```python
from build123d import *

# Parameters (mm, degrees)
SKETCH1_W                    = 200
SKETCH1_H                    = 70
BOSS_EXTRUDE1_DEPTH          = 150
CONVERT_SOLID1_START         = 1.36
CONVERT_SOLID1_DEPTH         = 197.28
CONVERT_SOLID1_START_2       = -1
CONVERT_SOLID1_2_DEPTH       = 202
CONVERT_SOLID1_3_DEPTH       = 2.184264069
CONVERT_SOLID1_START_3       = 198.815735931
CONVERT_SOLID1_4_DEPTH       = 2.184264069
CONVERT_SOLID1_START_4       = 1.184264069
CONVERT_SOLID1_5_DEPTH       = 197.631471862
CONVERT_SOLID1_6_DEPTH       = 0.175735931
CONVERT_SOLID1_START_5       = 198.64
CONVERT_SOLID1_7_DEPTH       = 0.175735931
CONVERT_SOLID1_START_6       = -68.815735931
CONVERT_SOLID1_8_DEPTH       = 67.631471862
CONVERT_SOLID1_9_DEPTH       = 0.175735931
CONVERT_SOLID1_START_7       = -1.36
CONVERT_SOLID1_10_DEPTH      = 0.175735931
EDGE_FLANGE1_STRIP_W         = 4.24
EDGE_FLANGE1_STRIP_H         = 0.76
EDGE_FLANGE1_STRIP_CUT_DEPTH = 148.269865
EDGE_FLANGE1_DEPTH           = 148.269865
MIRROR2_COPY_1_SKETCH_W      = 4.24
MIRROR2_COPY_1_SKETCH_H      = 0.76
MIRROR2_COPY_1_DEPTH         = 148.269865
MIRROR2_COPY_2_DEPTH         = 148.269865


with BuildPart() as part:
    # Sketch1 → Boss-Extrude1 (new body)
    with BuildSketch(Plane(origin=(0, 0, 0), x_dir=(1, 0, 0), z_dir=(0, 1, 0))):
        with Locations((100, 35)):
            Rectangle(SKETCH1_W, SKETCH1_H)
    extrude(amount=BOSS_EXTRUDE1_DEPTH)

    # Convert-Solid1: read off the stored shape, not the designer's step
    # Convert-Solid1 outline → Convert-Solid1 (cut)
    with BuildSketch(Plane.YZ.offset(CONVERT_SOLID1_START)):
        with BuildLine():
            Line((150, -0.76), (1.36, -0.76))
            ThreePointArc((1.36, -0.76), (0.935735931, -0.935735931), (0.76, -1.36))
            Line((0.76, -1.36), (0.76, -68.64))
            ThreePointArc((0.76, -68.64), (0.935735931, -69.064264069), (1.36, -69.24))
            Line((1.36, -69.24), (150, -69.24))
            Line((150, -69.24), (150, -0.76))
        make_face()
    extrude(amount=CONVERT_SOLID1_DEPTH, mode=Mode.SUBTRACT)

    # Convert-Solid1 2 outline → Convert-Solid1 2 (cut)
    with BuildSketch(Plane.YZ.offset(CONVERT_SOLID1_START_2)):
        with BuildLine():
            Line((0.76, -1.36), (1.730135, -1.36))
            Line((1.730135, -1.36), (1.730135, -1.184264069))
            Line((1.730135, -1.184264069), (150, -1.184264069))
            Line((150, -1.184264069), (150, -0.76))
            Line((150, -0.76), (1.36, -0.76))
            ThreePointArc((1.36, -0.76), (0.935735931, -0.935735931), (0.76, -1.36))
        make_face()
        with BuildLine():
            Line((1.730135, -68.64), (0.76, -68.64))
            ThreePointArc((0.76, -68.64), (0.935735931, -69.064264069), (1.36, -69.24))
            Line((1.36, -69.24), (150, -69.24))
            Line((150, -69.24), (150, -68.815735931))
            Line((150, -68.815735931), (1.730135, -68.815735931))
            Line((1.730135, -68.815735931), (1.730135, -68.64))
        make_face()
    extrude(amount=CONVERT_SOLID1_2_DEPTH, mode=Mode.SUBTRACT)

    # Convert-Solid1 3 outline → Convert-Solid1 3 (cut)
    with BuildSketch(Plane.YZ.offset(CONVERT_SOLID1_START_2)):
        with BuildLine():
            Line((150, -69.24), (1.36, -69.24))
            ThreePointArc((1.36, -69.24), (0.935735931, -69.064264069), (0.76, -68.64))
            Line((0.76, -68.64), (0, -68.64))
            Line((0, -68.64), (0, -70))
            Line((0, -70), (150, -70))
            Line((150, -70), (150, -69.24))
        make_face()
        with BuildLine():
            Line((0, 0), (0, -1.36))
            Line((0, -1.36), (0.76, -1.36))
            ThreePointArc((0.76, -1.36), (0.935735931, -0.935735931), (1.36, -0.76))
            Line((1.36, -0.76), (150, -0.76))
            Line((150, -0.76), (150, 0))
            Line((150, 0), (0, 0))
        make_face()
    extrude(amount=CONVERT_SOLID1_3_DEPTH, mode=Mode.SUBTRACT)

    # Convert-Solid1 4 outline → Convert-Solid1 4 (cut)
    with BuildSketch(Plane.YZ.offset(CONVERT_SOLID1_START_3)):
        with BuildLine():
            Line((150, -69.24), (1.36, -69.24))
            ThreePointArc((1.36, -69.24), (0.935735931, -69.064264069), (0.76, -68.64))
            Line((0.76, -68.64), (0, -68.64))
            Line((0, -68.64), (0, -70))
            Line((0, -70), (150, -70))
            Line((150, -70), (150, -69.24))
        make_face()
        with BuildLine():
            Line((0, 0), (0, -1.36))
            Line((0, -1.36), (0.76, -1.36))
            ThreePointArc((0.76, -1.36), (0.935735931, -0.935735931), (1.36, -0.76))
            Line((1.36, -0.76), (150, -0.76))
            Line((150, -0.76), (150, 0))
            Line((150, 0), (0, 0))
        make_face()
    extrude(amount=CONVERT_SOLID1_4_DEPTH, mode=Mode.SUBTRACT)

    # Convert-Solid1 5 outline → Convert-Solid1 5 (cut)
    with BuildSketch(Plane.YZ.offset(CONVERT_SOLID1_START_4)):
        with BuildLine():
            Line((0, -70), (1.36, -70))
            ThreePointArc((1.36, -70), (0.398334778, -69.601665222), (0, -68.64))
            Line((0, -68.64), (0, -70))
        make_face()
        with BuildLine():
            Line((0, 0), (0, -1.36))
            ThreePointArc((0, -1.36), (0.398334778, -0.398334778), (1.36, 0))
            Line((1.36, 0), (0, 0))
        make_face()
    extrude(amount=CONVERT_SOLID1_5_DEPTH, mode=Mode.SUBTRACT)

    # Convert-Solid1 6 outline → Convert-Solid1 6 (cut)
    with BuildSketch(Plane.YZ.offset(CONVERT_SOLID1_START_4)):
        with BuildLine():
            Line((1.730135, -70), (1.730135, -69.24))
            Line((1.730135, -69.24), (1.36, -69.24))
            ThreePointArc((1.36, -69.24), (0.935735931, -69.064264069), (0.76, -68.64))
            Line((0.76, -68.64), (0, -68.64))
            ThreePointArc((0, -68.64), (0.398334778, -69.601665222), (1.36, -70))
            Line((1.36, -70), (1.730135, -70))
        make_face()
        with BuildLine():
            ThreePointArc((1.36, 0), (0.398334778, -0.398334778), (0, -1.36))
            Line((0, -1.36), (0.76, -1.36))
            ThreePointArc((0.76, -1.36), (0.935735931, -0.935735931), (1.36, -0.76))
            Line((1.36, -0.76), (1.730135, -0.76))
            Line((1.730135, -0.76), (1.730135, 0))
            Line((1.730135, 0), (1.36, 0))
        make_face()
    extrude(amount=CONVERT_SOLID1_6_DEPTH, mode=Mode.SUBTRACT)

    # Convert-Solid1 7 outline → Convert-Solid1 7 (cut)
    with BuildSketch(Plane.YZ.offset(CONVERT_SOLID1_START_5)):
        with BuildLine():
            Line((1.730135, -70), (1.730135, -69.24))
            Line((1.730135, -69.24), (1.36, -69.24))
            ThreePointArc((1.36, -69.24), (0.935735931, -69.064264069), (0.76, -68.64))
            Line((0.76, -68.64), (0, -68.64))
            ThreePointArc((0, -68.64), (0.398334778, -69.601665222), (1.36, -70))
            Line((1.36, -70), (1.730135, -70))
        make_face()
        with BuildLine():
            ThreePointArc((1.36, 0), (0.398334778, -0.398334778), (0, -1.36))
            Line((0, -1.36), (0.76, -1.36))
            ThreePointArc((0.76, -1.36), (0.935735931, -0.935735931), (1.36, -0.76))
            Line((1.36, -0.76), (1.730135, -0.76))
            Line((1.730135, -0.76), (1.730135, 0))
            Line((1.730135, 0), (1.36, 0))
        make_face()
    extrude(amount=CONVERT_SOLID1_7_DEPTH, mode=Mode.SUBTRACT)

    # Convert-Solid1 8 outline → Convert-Solid1 8 (cut)
    with BuildSketch(Plane.XY.offset(CONVERT_SOLID1_START_6)):
        with BuildLine():
            Line((0, 0), (1.36, 0))
            ThreePointArc((1.36, 0), (0.398334778, 0.398334778), (0, 1.36))
            Line((0, 1.36), (0, 0))
        make_face()
        with BuildLine():
            ThreePointArc((200, 1.36), (199.601665222, 0.398334778), (198.64, 0))
            Line((198.64, 0), (200, 0))
            Line((200, 0), (200, 1.36))
        make_face()
        with BuildLine():
            ThreePointArc((0.76, 1.36), (0.935735931, 0.935735931), (1.36, 0.76))
            Line((1.36, 0.76), (1.36, 150))
            Line((1.36, 150), (0.76, 150))
            Line((0.76, 150), (0.76, 1.36))
        make_face()
        with BuildLine():
            ThreePointArc((198.64, 0.76), (199.064264069, 0.935735931), (199.24, 1.36))
            Line((199.24, 1.36), (199.24, 150))
            Line((199.24, 150), (198.64, 150))
            Line((198.64, 150), (198.64, 0.76))
        make_face()
    extrude(amount=CONVERT_SOLID1_8_DEPTH, mode=Mode.SUBTRACT)

    # Convert-Solid1 9 outline → Convert-Solid1 9 (cut)
    with BuildSketch(Plane.XY.offset(CONVERT_SOLID1_START_6)):
        with BuildLine():
            ThreePointArc((0, 1.36), (0.398334778, 0.398334778), (1.36, 0))
            Line((1.36, 0), (1.36, 0.76))
            ThreePointArc((1.36, 0.76), (0.935735931, 0.935735931), (0.76, 1.36))
            Line((0.76, 1.36), (0.76, 1.730135))
            Line((0.76, 1.730135), (0, 1.730135))
            Line((0, 1.730135), (0, 1.36))
        make_face()
        with BuildLine():
            Line((198.64, 0.76), (198.64, 0))
            ThreePointArc((198.64, 0), (199.601665222, 0.398334778), (200, 1.36))
            Line((200, 1.36), (200, 1.730135))
            Line((200, 1.730135), (199.24, 1.730135))
            Line((199.24, 1.730135), (199.24, 1.36))
            ThreePointArc((199.24, 1.36), (199.064264069, 0.935735931), (198.64, 0.76))
        make_face()
    extrude(amount=CONVERT_SOLID1_9_DEPTH, mode=Mode.SUBTRACT)

    # Convert-Solid1 10 outline → Convert-Solid1 10 (cut)
    with BuildSketch(Plane.XY.offset(CONVERT_SOLID1_START_7)):
        with BuildLine():
            ThreePointArc((0, 1.36), (0.398334778, 0.398334778), (1.36, 0))
            Line((1.36, 0), (1.36, 0.76))
            ThreePointArc((1.36, 0.76), (0.935735931, 0.935735931), (0.76, 1.36))
            Line((0.76, 1.36), (0.76, 1.730135))
            Line((0.76, 1.730135), (0, 1.730135))
            Line((0, 1.730135), (0, 1.36))
        make_face()
        with BuildLine():
            Line((198.64, 0.76), (198.64, 0))
            ThreePointArc((198.64, 0), (199.601665222, 0.398334778), (200, 1.36))
            Line((200, 1.36), (200, 1.730135))
            Line((200, 1.730135), (199.24, 1.730135))
            Line((199.24, 1.730135), (199.24, 1.36))
            ThreePointArc((199.24, 1.36), (199.064264069, 0.935735931), (198.64, 0.76))
        make_face()
    extrude(amount=CONVERT_SOLID1_10_DEPTH, mode=Mode.SUBTRACT)

    # Edge-Flange1: sheet metal written as solids
    # Edge-Flange1 strip (on a plane across the edge) → Edge-Flange1 strip cut (cut)
    with BuildSketch(Plane(origin=(199.24, 1.730135, -1.184264069), x_dir=(0, 0, -1), z_dir=(0, 1, 0))):
        with Locations((-0.76, -0.38)):
            Rectangle(EDGE_FLANGE1_STRIP_W, EDGE_FLANGE1_STRIP_H)
    edge_flange1_strip_cut = extrude(amount=EDGE_FLANGE1_STRIP_CUT_DEPTH, mode=Mode.SUBTRACT)

    # Edge-Flange1 section (on a plane across the edge) → Edge-Flange1 (add)
    with BuildSketch(Plane(origin=(199.24, 1.730135, -1.184264069), x_dir=(0, 0, -1), z_dir=(0, 1, 0))):
        with BuildLine():
            Line((0, 0.6), (0, 15))
            Line((0, 15), (0.76, 15))
            Line((0.76, 15), (0.76, 0.6))
            ThreePointArc((0.76, 0.6), (0.935735931, 0.175735931), (1.36, 0))
            Line((1.36, 0), (1.36, -0.76))
            ThreePointArc((1.36, -0.76), (0.398334778, -0.361665222), (0, 0.6))
        make_face()
    edge_flange1 = extrude(amount=EDGE_FLANGE1_DEPTH)

    # Mirror1: Edge-Flange1 strip cut, Edge-Flange1 across plane
    add(edge_flange1_strip_cut.mirror(Plane(origin=(100, 0, 0), x_dir=(0, 0, 1), z_dir=(1, 0, 0))), mode=Mode.SUBTRACT)
    add(edge_flange1.mirror(Plane(origin=(100, 0, 0), x_dir=(0, 0, 1), z_dir=(1, 0, 0))))

    # Mirror2: Edge-Flange1 strip cut, Edge-Flange1 across plane
    add(edge_flange1_strip_cut.mirror(Plane.XY.offset(-35)), mode=Mode.SUBTRACT)
    add(edge_flange1.mirror(Plane.XY.offset(-35)))

    # Mirror2 copy 1 sketch → Mirror2 copy 1 (cut)
    with BuildSketch(Plane(origin=(0.76, 1.730135, -68.815735931), x_dir=(0, 0, 1), z_dir=(0, 1, 0))):
        with Locations((-0.76, -0.38)):
            Rectangle(MIRROR2_COPY_1_SKETCH_W, MIRROR2_COPY_1_SKETCH_H)
    extrude(amount=MIRROR2_COPY_1_DEPTH, mode=Mode.SUBTRACT)

    # Mirror2 copy 2 sketch → Mirror2 copy 2 (add)
    with BuildSketch(Plane(origin=(0.76, 1.730135, -68.815735931), x_dir=(0, 0, 1), z_dir=(0, 1, 0))):
        with BuildLine():
            Line((0, 0.6), (0, 15))
            Line((0, 15), (0.76, 15))
            Line((0.76, 15), (0.76, 0.6))
            ThreePointArc((0.76, 0.6), (0.935735931, 0.175735931), (1.36, 0))
            Line((1.36, 0), (1.36, -0.76))
            ThreePointArc((1.36, -0.76), (0.398334778, -0.361665222), (0, 0.6))
        make_face()
    extrude(amount=MIRROR2_COPY_2_DEPTH)


solid = part.part
```
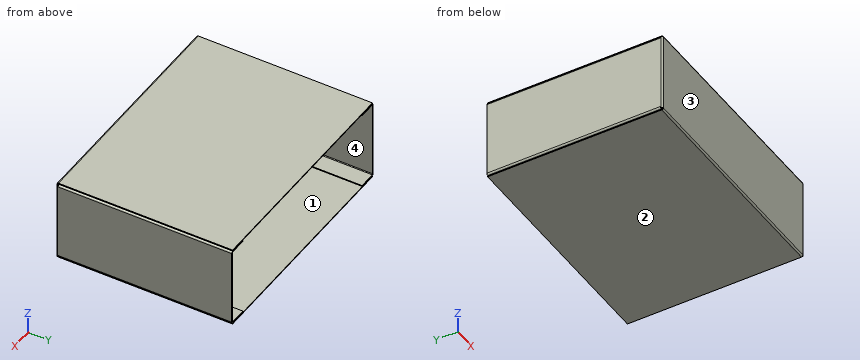
Check sheet for the modelled part. Datum: model origin and axes. Units: mm. Face numbers are marked on the shaded views. Round coordinates to 2 decimals unless told otherwise and drop trailing zeros. Order: outer loops, then holes, each group sorted by start corner. A loop starts at its lowest first (then second) coordinate and runs counter-clockwise, first axis right, second up. Notation, with made-up numbers: (-1.5, 40.5) - (20.5, 40.5) arc R18 ccw to (20.5, 59.5) - close; hole circle Ø10 at (-18, 51). An arc over 180 degrees is marked (long way). Answer as CSV lines item,"result". Start each with the question number.
1) Section check C-C (x = 23). Record the cut outline in (y, z), then the cut area to 3 significant figures.
2) Section check B-B (z = -54). Record the cut outline in (x, y), then the cut area to 3 significant figures.
3) Depth check by flat-ended pin: pin 1 (16 mm diameter, centred on x = 188, y = 104.5, fed in from +Z); pin 2 (10 mm diameter, centred on x = 105.5, z = -29.5, fed in from +Y); pin 3 (1.1 mm diameter, centred on x = 199.5, y = 1, fed in from +Z); pin 4 (1.1 mm diameter, centred on y = 0.5, z = -69, fed in from +X). Enter the tip coordinate at first touch or a pass-through.
4) Draft check along Z on the marked faces 1, 2, 3 and 4. Enter one of: +Z half, -Z half, draft (parallel to the pull), parting line (faces both ways), or undercut.
5) Section check A-A (y = 82.5). Give the number of separate pieces and of enclosed holes in the cut face, then the cut area to 3 significant figures.
6) Scan lines: probe 1 along Z at (x, y) = (8, 60); probe 2 along X at (y, z) = (86, -38.5); probe 3 along Z at (x, y) = (36, 118.5). Record each from-to range of solid material in increasing order.
Determined:
1,outline,"(0, -68.64) arc R1.36 ccw to (1.36, -70) - (150, -70) - (150, -69.24) - (1.36, -69.24) arc R0.6 cw to (0.76, -68.64) - (0.76, -1.36) arc R0.6 cw to (1.36, -0.76) - (150, -0.76) - (150, 0) - (1.36, 0) arc R1.36 ccw to (0, -1.36) - close"
1,area,"279 mm^2"
2,outline,"(0, 1.36) arc R1.36 ccw to (1.36, 0) - (198.64, 0) arc R1.36 ccw to (200, 1.36) - (200, 150) - (199.24, 150) - (199.24, 1.36) arc R0.6 cw to (198.64, 0.76) - (1.36, 0.76) arc R0.6 cw to (0.76, 1.36) - (0.76, 150) - (0, 150) - close"
2,area,"378 mm^2"
3,pin 1,"z = 0"
3,pin 2,"y = 0.76"
3,pin 3,"z = -1.36"
3,pin 4,"x = 199.93"
4,face 1,"undercut"
4,face 2,"-Z half"
4,face 3,"draft"
4,face 4,"undercut"
5,separate pieces,"4"
5,enclosed holes,"0"
5,area,"448 mm^2"
6,probe 1,"-70 to -69.24, -68.82 to -68.06, -1.94 to -1.18, -0.76 to 0"
6,probe 2,"0 to 0.76, 199.24 to 200"
6,probe 3,"-70 to -69.24, -0.76 to 0"
